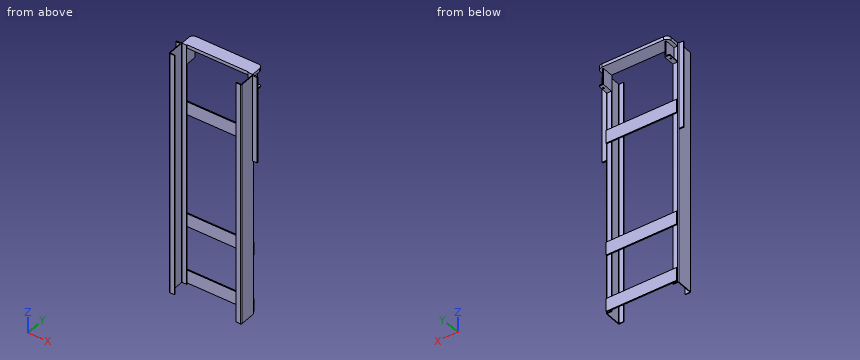
```python
from build123d import *

# Parameters (mm, degrees)
EXTRUDE_THIN1_DEPTH  = 1400
SKETCH2_W            = 50
SKETCH2_H            = 12.5
BOSS_EXTRUDE1_DEPTH  = 1000
BOSS_EXTRUDE2_DEPTH  = 38
SKETCH4_W            = 806
SKETCH4_H            = 150
BOSS_EXTRUDE3_DEPTH  = 12.5
LPATTERN1_COUNT      = 2
LPATTERN1_PITCH      = 660
LPATTERN2_COUNT      = 2
LPATTERN2_PITCH      = 1970
SKETCH5_W            = 12.5
SKETCH5_H            = 127
BOSS_EXTRUDE4_DEPTH  = 175
SKETCH6_W            = 53
SKETCH6_H            = 127
SKETCH6_R            = 8.75
BOSS_EXTRUDE5_DEPTH  = 12.5
FILLET1_R            = 12.5
FILLET1_OF_MIRROR3_R = 12.5


with BuildPart() as part:
    # Sketch1 → Extrude-Thin1 (new, symmetric)
    with BuildSketch(Plane.XY):
        with BuildLine():
            Line((350, 100), (403, 100))
            ThreePointArc((403, 100), (410.071067812, 97.071067812), (413, 90))
            Line((413, 90), (413, -90))
            ThreePointArc((413, -90), (410.071067812, -97.071067812), (403, -100))
            Line((403, -100), (350, -100))
            Line((350, -100), (350, -92.5))
            Line((350, -92.5), (403, -92.5))
            ThreePointArc((403, -92.5), (404.767766953, -91.767766953), (405.5, -90))
            Line((405.5, -90), (405.5, 90))
            ThreePointArc((405.5, 90), (404.767766953, 91.767766953), (403, 92.5))
            Line((403, 92.5), (350, 92.5))
            Line((350, 92.5), (350, 100))
        make_face()
    extrude(amount=EXTRUDE_THIN1_DEPTH, both=True)

    # Sketch2 → Boss-Extrude1 (add)
    with BuildSketch(Plane.XY.offset(1400)):
        with Locations((438, 83.75)):
            Rectangle(SKETCH2_W, SKETCH2_H)
    extrude(amount=-BOSS_EXTRUDE1_DEPTH)


with BuildPart() as body_2:
    # Mirror2: mirrored copy
    add(part.part.mirror(Plane(origin=(0, 0, 0), x_dir=(0, 0, 1), z_dir=(1, 0, 0))))


with BuildPart() as part_1:
    add(part.part)

    add(body_2.part)  # Boss-Extrude2 merges body 2
    # Sketch3 → Boss-Extrude2 (add)
    with BuildSketch(Plane.XY.offset(1400)):
        with BuildLine():
            Line((-403, 100), (403, 100))
            Line((403, 100), (403, 200))
            ThreePointArc((403, 200), (388.355339059, 235.355339059), (353, 250))
            Line((353, 250), (-353, 250))
            ThreePointArc((-353, 250), (-388.355339059, 235.355339059), (-403, 200))
            Line((-403, 200), (-403, 100))
        make_face()
    extrude(amount=-BOSS_EXTRUDE2_DEPTH)

    # Sketch4 → Boss-Extrude3 (add)
    with BuildSketch(Plane(origin=(0, 100, 0), x_dir=(1, 0, 0), z_dir=(0, 1, 0))):
        with Locations((0, 1312.5)):
            Rectangle(SKETCH4_W, SKETCH4_H)
    boss_extrude3 = extrude(amount=BOSS_EXTRUDE3_DEPTH)

    # LPattern1: Boss-Extrude3 ×2
    with Locations(*[(0, 0, i * LPATTERN1_PITCH) for i in range(1, LPATTERN1_COUNT)]):
        add(boss_extrude3)

    # LPattern2: Boss-Extrude3 ×2
    with Locations(*[(0, 0, i * LPATTERN2_PITCH) for i in range(1, LPATTERN2_COUNT)]):
        add(boss_extrude3)

    # Sketch5 → Boss-Extrude4 (add)
    with BuildSketch(Plane(origin=(0, 0, 1362), x_dir=(-1, 0, 0), z_dir=(0, 0, -1))):
        with Locations((-356.25, 163.5)):
            Rectangle(SKETCH5_W, SKETCH5_H)
    boss_extrude4 = extrude(amount=BOSS_EXTRUDE4_DEPTH)

    # Sketch6 → Boss-Extrude5 (add)
    with BuildSketch(Plane(origin=(0, 0, 1187), x_dir=(-1, 0, 0), z_dir=(0, 0, -1))):
        with Locations((-376.5, 163.5)):
            Rectangle(SKETCH6_W, SKETCH6_H)
        with Locations((-384, 182)):
            Circle(SKETCH6_R, mode=Mode.SUBTRACT)
    boss_extrude5 = extrude(amount=BOSS_EXTRUDE5_DEPTH)

    # Fillet1
    fillet1_edges = [part_1.edges().sort_by_distance(p)[0] for p in [
        (403, 227, 1180.75),
    ]]
    fillet(fillet1_edges, radius=FILLET1_R)

    # Mirror3: Boss-Extrude4, Boss-Extrude5 across plane
    add(boss_extrude4.mirror(Plane(origin=(0, 0, 0), x_dir=(0, 0, 1), z_dir=(1, 0, 0))))
    add(boss_extrude5.mirror(Plane(origin=(0, 0, 0), x_dir=(0, 0, 1), z_dir=(1, 0, 0))))

    # Fillet1 of Mirror3
    fillet1_of_mirror3_edges = [part_1.edges().sort_by_distance(p)[0] for p in [
        (-403, 227, 1180.75),
    ]]
    fillet(fillet1_of_mirror3_edges, radius=FILLET1_OF_MIRROR3_R)


solid = part_1.part
```
Build history of the part. All positions in model axes, mm. Give positions to 0.01 mm unless a question says otherwise; leave off trailing zeros. Loops run counter-clockwise (first coordinate to the right, second up) from the corner with the lowest first, then second, coordinate; pieces in that order, holes last. Notation, with made-up numbers: (-37, 8.5) -> (-24, 8.5) arc R12 ccw to (-24, 26.5) -> close; hole circle Ø5 at (48, -39.75). An arc over 180 degrees is marked (long way). One line per question, with ' | ' between items. Start each with the question number.
1) Pin check, flat tips, straight feed: pin 1 (10 mm diameter, centred on x = 146, y = 106.5, fed in from -Z); pin 2 (11.5 mm diameter, centred on x = -133, z = 1390.5, fed in from -Y); pin 3 (6 mm diameter, centred on x = 385.5, z = -1396, fed in from +Y). Stop position of each tip, or through.
2) Cut at A-A (x = -157.5). Give the cut face in (y, z), plus the area to 3 significant figures.
3) Probe L1, parallel to Y at x = 384, z = 1179; L2, parallel to X at y = 75, z = 1223; L3, parallel to Y at x = 361, z = -131. List the from-to ranges inside material, lowest first.
4) Cut at C-C (z = -234.5). Give the cut face in (x, y), plus the area to 3 significant figures.
5) Cut at B-B (y = -16.5). Give the cut face in (x, z), plus the area to 3 significant figures.
Return value:
1) pin 1: z = -1387.5 | pin 2: y = 100 | pin 3: y = 100
2) outline: (100, -1387.5) -> (112.5, -1387.5) -> (112.5, -1237.5) -> (100, -1237.5) -> close; (100, -727.5) -> (112.5, -727.5) -> (112.5, -577.5) -> (100, -577.5) -> close; (100, 582.5) -> (112.5, 582.5) -> (112.5, 732.5) -> (100, 732.5) -> close; (100, 1362) -> (250, 1362) -> (250, 1400) -> (100, 1400) -> close | area: 11,300 mm^2
3) L1: -100 to -92.5, 92.5 to 173.25, 190.75 to 227 | L2: -413 to -405.5, 405.5 to 413 | L3: -100 to -92.5, 92.5 to 100
4) outline: (-413, -90) arc R10 ccw to (-403, -100) -> (-350, -100) -> (-350, -92.5) -> (-403, -92.5) arc R2.5 cw to (-405.5, -90) -> (-405.5, 90) arc R2.5 cw to (-403, 92.5) -> (-350, 92.5) -> (-350, 100) -> (-403, 100) arc R10 ccw to (-413, 90) -> close; (350, -100) -> (403, -100) arc R10 ccw to (413, -90) -> (413, 90) arc R10 ccw to (403, 100) -> (350, 100) -> (350, 92.5) -> (403, 92.5) arc R2.5 cw to (405.5, 90) -> (405.5, -90) arc R2.5 cw to (403, -92.5) -> (350, -92.5) -> close | area: 4,580 mm^2
5) outline: (-413, -1400) -> (-405.5, -1400) -> (-405.5, 1400) -> (-413, 1400) -> close; (405.5, -1400) -> (413, -1400) -> (413, 1400) -> (405.5, 1400) -> close | area: 42,000 mm^2
